from build123d import *

# Parameters (mm, degrees)
SKETCH1_W           = 23
SKETCH1_H           = 70.95
BOSS_EXTRUDE1_DEPTH = 200
SKETCH2_W           = 19
SKETCH2_H           = 70.95
CUT_EXTRUDE1_DEPTH  = 204.447107684
SKETCH3_W           = 70.95
SKETCH3_H           = 1
BOSS_EXTRUDE2_DEPTH = 19


with BuildPart() as part:
    # Sketch1 → Boss-Extrude1 (new body)
    with BuildSketch(Plane(origin=(0, 0, 0), x_dir=(1, 0, 0), z_dir=(0, 1, 0))):
        Rectangle(SKETCH1_W, SKETCH1_H)
    extrude(amount=BOSS_EXTRUDE1_DEPTH)

    # Sketch2 → Cut-Extrude1 (cut, through all)
    with BuildSketch(Plane(origin=(0, 200, 0), x_dir=(1, 0, 0), z_dir=(0, 1, 0))):
        with Locations((-2, 0)):
            Rectangle(SKETCH2_W, SKETCH2_H)
    extrude(amount=-CUT_EXTRUDE1_DEPTH, mode=Mode.SUBTRACT)

    # Sketch3 → Boss-Extrude2 (add)
    with BuildSketch(Plane.ZY.offset(-7.5)):
        with Locations((0, 80)):
            Rectangle(SKETCH3_W, SKETCH3_H)
        with Locations((0, 120)):
            Rectangle(SKETCH3_W, SKETCH3_H)
    extrude(amount=BOSS_EXTRUDE2_DEPTH)


solid = part.part
Part model, mm, in its own coordinate system. A direction names the side the tool comes from. Coordinates: 2 decimals unless noted, no trailing zeros. Write each loop counter-clockwise with the first axis right and the second up, starting at its lowest first coordinate (ties: lowest second). Pieces come first, ordered by that corner, then holes. Notation, with made-up numbers: M 47.25,61 L 79.25,61 A14 ccw 79.25,65 Z; hole C 22.25,-31.5 d1. An arc over 180 degrees is marked long. Return JSON: item names as keys, results as strings.
1. Probe L1, parallel to Y at x = -2, z = -25.5; L2, parallel to X at y = 88, z = 20. List the from-to ranges inside material, lowest first.
Determined:
{"L1": "79.5 to 80.5, 119.5 to 120.5", "L2": "7.5 to 11.5"}
2. Saw through at A-A, the plane x = 5. Write the cut outline in (y, z) (3 decimals).
Determined:
{"outline": "M 79.5,-35.475 L 80.5,-35.475 L 80.5,35.475 L 79.5,35.475 Z; M 119.5,-35.475 L 120.5,-35.475 L 120.5,35.475 L 119.5,35.475 Z"}
3. 3-axis set-ups, long thin cutter, end or side, ignore diameter. For faces 4 (the face through (7.5, 161, 0)), 5 (the face through (-2, 79.5, 0)), 6 (the face through (7.5, 100, 0)): which of +Z, -Z, +X, -X, +Y, -Y reach the whole face in a straight line?
Determined:
{"face 4": "+Z, -Z, -X, +Y", "face 5": "+Z, -Z, -X, -Y", "face 6": "+Z, -Z, -X"}
4. Saw through at C-C, the plane y = 153. Write the cut outline in (x, z) (3 decimals).
Determined:
{"outline": "M 7.5,-35.475 L 11.5,-35.475 L 11.5,35.475 L 7.5,35.475 Z"}
5. Flat gauge pins, fed straight in: pin 1 Ø10 at (x, z) = (-3.5, -0.5) entering from +Y; pin 2 Ø5.5 at (x, z) = (-3, 1) entering from -Y; pin 3 Ø4 at (y, z) = (27.5, -7) entering from -X. Where does each tip first touch, or does it go through?
Determined:
{"pin 1": "y = 120.5", "pin 2": "y = 79.5", "pin 3": "x = 7.5"}
6. Saw through at B-B, the plane z = -1.5. Write the cut outline in (x, y), then the cut area to 3 significant figures.
Determined:
{"outline": "M -11.5,79.5 L 7.5,79.5 L 7.5,0 L 11.5,0 L 11.5,200 L 7.5,200 L 7.5,120.5 L -11.5,120.5 L -11.5,119.5 L 7.5,119.5 L 7.5,80.5 L -11.5,80.5 Z", "area": "838 mm²"}
7. Pull direction Y, two halves, no side cores. Call faces 1 (the face through (-2, 80.5, 0)), 2 (the face through (11.5, 99, 0)), 3 (the face through (9, 0, 0)): pulls with the +Y half, pulls with the -Y half, needs draft (parallel to the pull), parting line crosses it, or undercut.
Determined:
{"face 1": "undercut", "face 2": "needs draft", "face 3": "pulls with the -Y half"}
